Verification items for the finished model (mm, model axes). Face numbers are marked on the shaded views. A direction names the side the tool comes from. Coordinates: 2 decimals unless noted, no trailing zeros. Loops run counter-clockwise (first coordinate to the right, second up) from the corner with the lowest first, then second, coordinate; pieces in that order, holes last.
Q1. Material ranges on probe 1 along X at (y, z) = (20, 12.25); probe 2 along Y at (x, z) = (-5, -3); probe 3 along X at (y, z) = (27.5, 10.75), recorded low to high.
Q2. Access from +Z, -Z, +X, -X, +Y, -Y to the whole of each face (thin tool, end or side, straight path). Record for the marked faces 4, 5, 6 and 7.
Q3. Go/stop test with flat-tipped pins: P1, Ø5.5, axis at x = 13.5, z = -3, coming from the +Y side; P2, Ø5, axis at y = 21.8, z = 14.85, coming from the -X side; P3, Ø8, axis at x = 9, y = 17.5, coming from the +Z side (3 decimals). Record where each tip stops, or that it passes through.
Q4. Sectioned sample at A-A (x = -8). Enter the section's corners in (y, z), then the cut area to 3 significant figures.
Q5. Mould release check, pull along Y, two halves, no side actions. Record for the marked faces 1, 2 and 3: +Y half, -Y half, draft (parallel to the pull), parting line (faces both ways), or undercut.
Q6. Sectioned sample at C-C (y = 17). Count the separate pieces of the cut face and the enclosed holes in it, then the cut area to 3 significant figures.
Q7. Sectioned sample at B-B (y = 4.3). Enter the section's corners in (x, z), then the cut area to 3 significant figures.
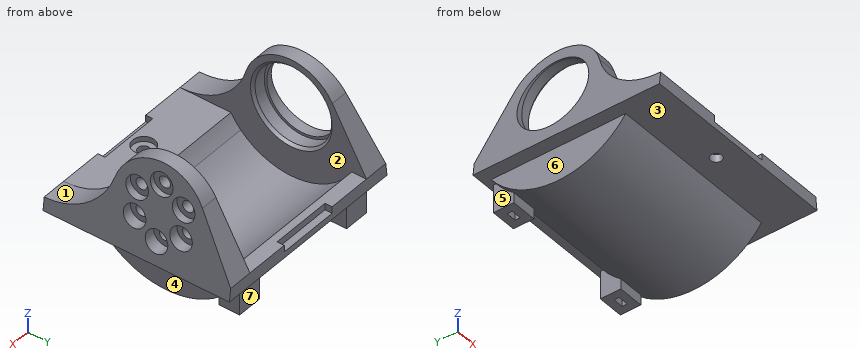
```python
from build123d import *

# Parameters (mm, degrees)
SKETCH_1_W                   = 39.5
SKETCH_1_H                   = 36.5
EXTRUDE_1_DEPTH              = 2.5
EXTRUDE_START                = -2.6
EXTRUDE_2_DEPTH              = 34
EXTRUDE_START_2              = 14.6
EXTRUDE_3_DEPTH              = 5.15
SKETCH_4_W                   = 5
SKETCH_4_H                   = 4
EXTRUDE_4_DEPTH              = 5.5
CUT_EXTRUDE_1_REACH          = 50.117
CUT_EXTRUDE_1_END_RADIUS     = 16.3
SKETCH_5_W                   = 2
SKETCH_5_H                   = 1
CUT_EXTRUDE_2_DEPTH          = 29.2
SKETCH_7_R                   = 7.5
CUT_EXTRUDE_3_DEPTH          = 2.8
SKETCH_8_R                   = 7
CUT_EXTRUDE_4_DEPTH          = 56.3867764
CHAMFER_1_SIZE               = 0.5
SKETCH_9_W                   = 12
SKETCH_9_H                   = 1.4
CUT_EXTRUDE_5_DEPTH          = 1.3
HOLE_WIZARD_M2_1_D           = 2.2
HOLE_WIZARD_M2_1_CBORE_D     = 4.3
HOLE_WIZARD_M2_1_CBORE_DEPTH = 1
SKETCH_10_W                  = 12
SKETCH_10_H                  = 1.4
CUT_EXTRUDE_6_DEPTH          = 1.3
PATTERN_CIRCULAR_1_COUNT     = 6
CUT_EXTRUDE_7_DEPTH          = 46.581081602
SKETCH_17_R                  = 13.8
CUT_EXTRUDE_8_DEPTH          = 29.2


with BuildPart() as part:
    # 草图1 → 凸台-拉伸1 (new body)
    with BuildSketch(Plane.XY):
        with Locations((0, 18.25)):
            Rectangle(SKETCH_1_W, SKETCH_1_H)
    extrude(amount=EXTRUDE_1_DEPTH)

    # 草图2 → 凸台-拉伸2 (add)
    with BuildSketch(Plane.ZY.offset(19.75).offset(EXTRUDE_START)):
        with BuildLine():
            Line((2.5, 7.127576887), (2.5, 36.472423113))
            ThreePointArc((2.5, 36.472423113), (1.216414342, 35.778751429), (0, 34.973078608))
            Line((0, 34.973078608), (0, 8.626921392))
            ThreePointArc((0, 8.626921392), (1.216414342, 7.821248571), (2.5, 7.127576887))
        make_face()
        with BuildLine():
            Line((0, 8.626921392), (0, 34.973078608))
            ThreePointArc((0, 34.973078608), (-6.7, 21.8), (0, 8.626921392))
        make_face()
    extrude(amount=-EXTRUDE_2_DEPTH)

    # 草图3 → 凸台-拉伸3 (add, through all)
    with BuildSketch(Plane(origin=(0, 0, 0), x_dir=(0, 0, -1), z_dir=(1, 0, 0)).offset(EXTRUDE_START_2)):
        with BuildLine():
            Line((-2.5, 36.5), (-14.183665706, 29.834457586))
            ThreePointArc((-14.183665706, 29.834457586), (-18.787148585, 20.723523862), (-12.202183107, 12.923562478))
            ThreePointArc((-12.202183107, 12.923562478), (-5.203778934, 8.073846044), (-2.5, 0))
            Line((-2.5, 0), (-2.5, 36.5))
        make_face()
    extrude_3 = extrude(amount=EXTRUDE_3_DEPTH)

    # 镜向1: 凸台-拉伸3 across plane
    add(extrude_3.mirror(Plane(origin=(0, 0, 0), x_dir=(0, 0, 1), z_dir=(1, 0, 0))))

    # 草图4 → 凸台-拉伸4 (add)
    with BuildSketch(Plane(origin=(0, 0, 0), x_dir=(-1, 0, 0), z_dir=(0, 0, -1))):
        with Locations((-13.4, 33.5)):
            Rectangle(SKETCH_4_W, SKETCH_4_H)
        with Locations((13.4, 33.5)):
            Rectangle(SKETCH_4_W, SKETCH_4_H)
    extrude(amount=EXTRUDE_4_DEPTH)

    # 切除-拉伸1: up to this cylinder (the profile starts outside it)
    cut_extrude_1_end = Plane(origin=(0, 21.8, 9.6), z_dir=(-1, 0, 0)) * Cylinder(CUT_EXTRUDE_1_END_RADIUS, 160.634, mode=Mode.PRIVATE)
    # 草图5 → 切除-拉伸1 (cut, up to the surface)
    with BuildSketch(Plane(origin=(0, 0, -5.5), x_dir=(-1, 0, 0), z_dir=(0, 0, -1)), mode=Mode.PRIVATE) as cut_extrude_1_sk1:
        with Locations((-13.4, 33.5)):
            Rectangle(SKETCH_5_W, SKETCH_5_H)
    cut_extrude_1_tool1 = extrude(cut_extrude_1_sk1.sketch, amount=-CUT_EXTRUDE_1_REACH, mode=Mode.PRIVATE) - cut_extrude_1_end
    add(cut_extrude_1_tool1.solids().sort_by_distance((13.4, 33.5, -5.5))[0], mode=Mode.SUBTRACT)
    # 草图5 → 切除-拉伸1 (cut, up to the surface)
    with BuildSketch(Plane(origin=(0, 0, -5.5), x_dir=(-1, 0, 0), z_dir=(0, 0, -1)), mode=Mode.PRIVATE) as cut_extrude_1_sk2:
        with Locations((13.4, 33.5)):
            Rectangle(SKETCH_5_W, SKETCH_5_H)
    cut_extrude_1_tool2 = extrude(cut_extrude_1_sk2.sketch, amount=-CUT_EXTRUDE_1_REACH, mode=Mode.PRIVATE) - cut_extrude_1_end
    add(cut_extrude_1_tool2.solids().sort_by_distance((-13.4, 33.5, -5.5))[0], mode=Mode.SUBTRACT)

    # 草图6 → 切除-拉伸2 (cut)
    with BuildSketch(Plane(origin=(-14.6, 0, 0), x_dir=(0, 0, -1), z_dir=(1, 0, 0))):
        with BuildLine():
            Line((0, 31.713626985), (0, 11.886373015))
            ThreePointArc((0, 11.886373015), (-23.4, 21.8), (0, 31.713626985))
        make_face()
    extrude(amount=CUT_EXTRUDE_2_DEPTH, mode=Mode.SUBTRACT)

    # 草图7 → 切除-拉伸3 (cut)
    with BuildSketch(Plane(origin=(-14.6, 0, 0), x_dir=(0, 0, -1), z_dir=(1, 0, 0))):
        with Locations((-9.6, 21.8)):
            Circle(SKETCH_7_R)
    extrude(amount=-CUT_EXTRUDE_3_DEPTH, mode=Mode.SUBTRACT)

    # 草图8 → 切除-拉伸4 (cut, through all)
    with BuildSketch(Plane(origin=(-17.4, 0, 0), x_dir=(0, 0, -1), z_dir=(1, 0, 0))):
        with Locations((-9.6, 21.8)):
            Circle(SKETCH_8_R)
    extrude(amount=-CUT_EXTRUDE_4_DEPTH, mode=Mode.SUBTRACT)

    # 倒角1
    chamfer_1_edges = [part.edges().sort_by_distance(p)[0] for p in [
        (-14.6, 21.8, 17.1),
    ]]
    chamfer(chamfer_1_edges, length=CHAMFER_1_SIZE)

    # 草图9 → 切除-拉伸5 (cut)
    with BuildSketch(Plane.XY.offset(2.5)):
        with Locations((0, 35.8)):
            Rectangle(SKETCH_9_W, SKETCH_9_H)
    extrude(amount=-CUT_EXTRUDE_5_DEPTH, mode=Mode.SUBTRACT)

    # M2 六角圆柱头螺钉的柱形沉头孔1 (through all)
    with Locations(Plane.XY.offset(2.5)):
        with Locations((0, 4.3)):
            CounterBoreHole(HOLE_WIZARD_M2_1_D / 2, HOLE_WIZARD_M2_1_CBORE_D / 2, HOLE_WIZARD_M2_1_CBORE_DEPTH)

    # 草图10 → 切除-拉伸6 (cut)
    with BuildSketch(Plane.XY.offset(2.5)):
        with Locations((0, 0.7)):
            Rectangle(SKETCH_10_W, SKETCH_10_H)
    extrude(amount=-CUT_EXTRUDE_6_DEPTH, mode=Mode.SUBTRACT)

    # 草图15 → M2 六角圆柱头螺钉的柱形沉头孔2 (revolve, cut)
    with BuildSketch(Plane(origin=(19.75, 21.8, 14.85), x_dir=(0, 0, -1), z_dir=(0, 1, 0))):
        Polygon((0, 0), (0, 7.860946681), (1.1, 7.2), (1.1, 2.65), (2.2, 2.65), (2.2, 0), align=None)
    hole_wizard_m2_2 = revolve(axis=Axis((26.1, 21.8, 14.85), (-1, 0, 0)), mode=Mode.SUBTRACT)

    # 阵列(圆周)1: M2 六角圆柱头螺钉的柱形沉头孔2 ×6 about axis
    pattern_circular_1_axis = Axis((0, 21.8, 9.6), (1, 0, 0))
    for i in range(1, PATTERN_CIRCULAR_1_COUNT):
        add(hole_wizard_m2_2.rotate(pattern_circular_1_axis, i * 360 / PATTERN_CIRCULAR_1_COUNT), mode=Mode.SUBTRACT)

    # 草图16 → 切除-拉伸7 (cut, through all)
    with BuildSketch(Plane(origin=(0, 36.5, 0), x_dir=(1, 0, 0), z_dir=(0, 1, 0))):
        Polygon((19.75, 0), (17.392084769, -18.85), (19.75, -18.85), align=None)
        Polygon((-17.392084769, -18.85), (-19.75, -18.85), (-19.75, 0), align=None)
    extrude(amount=-CUT_EXTRUDE_7_DEPTH, mode=Mode.SUBTRACT)

    # 草图17 → 切除-拉伸8 (cut)
    with BuildSketch(Plane(origin=(-14.6, 0, 0), x_dir=(0, 0, -1), z_dir=(1, 0, 0))):
        with Locations((-9.6, 21.8)):
            Circle(SKETCH_17_R)
    extrude(amount=CUT_EXTRUDE_8_DEPTH, mode=Mode.SUBTRACT)


solid = part.part
```
Geometry check:
1. probe 1: x = 14.6 to 18.22
1. probe 2: y = 11.46 to 16.17, 27.43 to 32.14
1. probe 3: x = 14.6 to 17.1
2. face 4: -Z, +X, +Y, -Y
2. face 5: -Z, -X, +Y
2. face 6: -Z, -X, +Y, -Y
2. face 7: -Z, +X, -X, +Y
3. P1: stops at y = 35.5
3. P2: stops at x = -17.71
3. P3: stops at z = -1.425
4. outline: (0, 0) - (8.63, 0) arc R16.3 ccw to (34.97, 0) - (36.5, 0) - (36.5, 2.5) - (33.63, 2.5) arc R13.8 cw to (9.97, 2.5) - (0, 2.5) - close
4. area: 103 mm2
5. face 1: -Y half
5. face 2: undercut
5. face 3: draft
6. separate pieces: 4
6. enclosed holes: 0
6. area: 180 mm2
7. outline: (-19.75, 0) - (-1.1, 0) - (-1.1, 1.5) - (-2.15, 1.5) - (-2.15, 2.5) - (-14.6, 2.5) - (-14.6, 3.21) - (-19.35, 3.21) - close; (1.1, 0) - (19.75, 0) - (19.35, 3.21) - (14.6, 3.21) - (14.6, 2.5) - (2.15, 2.5) - (2.15, 1.5) - (1.1, 1.5) - close
7. area: 97.2 mm2
